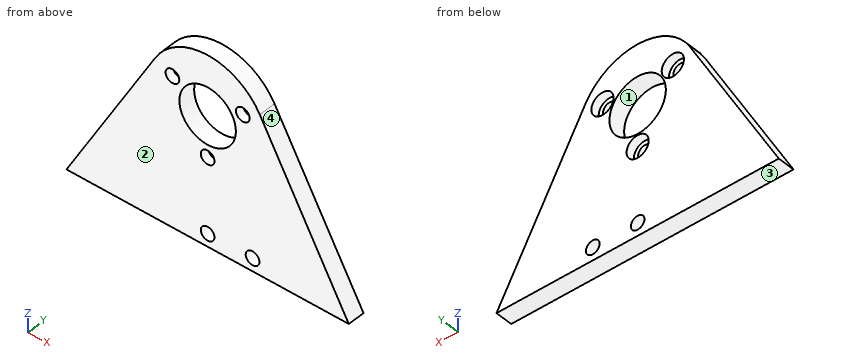
from build123d import *

# Parameters (mm, degrees)
EXTRUDE_1_DEPTH     = 4
SKETCH_3_R          = 1.6
SKETCH_3_R_2        = 6.6
CUT_EXTRUDE_3_DEPTH = 4
SKETCH_4_R          = 1.6
CUT_EXTRUDE_4_DEPTH = 4
SKETCH_5_R          = 2.6
CUT_EXTRUDE_6_DEPTH = 2


with BuildPart() as part:
    # 草图1 → 凸台-拉伸1 (new body)
    with BuildSketch(Plane(origin=(0, 0, 0), x_dir=(1, 0, 0), z_dir=(0, 1, 0))):
        with BuildLine():
            Line((33, 30), (12.193267422, -6.879260831))
            ThreePointArc((12.193267422, -6.879260831), (0, -14), (-12.193267422, -6.879260831))
            Line((-12.193267422, -6.879260831), (-33, 30))
            Line((-33, 30), (33, 30))
        make_face()
    extrude(amount=EXTRUDE_1_DEPTH)

    # 草图3 → 切除-拉伸3 (cut)
    with BuildSketch(Plane(origin=(0, 4, 0), x_dir=(1, 0, 0), z_dir=(0, 1, 0))):
        with Locations(Location((-8.227241336, -4.75, 0), (0, 0, 270))):
            Circle(SKETCH_3_R)
        with Locations(Location((8.227241336, -4.75, 0), (0, 0, 270))):
            Circle(SKETCH_3_R)
        with Locations(Location((0, 0, 0), (0, 0, 270))):
            Circle(SKETCH_3_R_2)
        with Locations(Location((0, 9.5, 0), (0, 0, 270))):
            Circle(SKETCH_3_R)
    extrude(amount=-CUT_EXTRUDE_3_DEPTH, mode=Mode.SUBTRACT)

    # 草图4 → 切除-拉伸4 (cut)
    with BuildSketch(Plane(origin=(0, 4, 0), x_dir=(1, 0, 0), z_dir=(0, 1, 0))):
        with Locations(Location((0, 27, 0), (0, 0, 270))):
            Circle(SKETCH_4_R)
        with Locations(Location((10.5, 27, 0), (0, 0, 270))):
            Circle(SKETCH_4_R)
    extrude(amount=-CUT_EXTRUDE_4_DEPTH, mode=Mode.SUBTRACT)

    # 草图5 → 切除-拉伸6 (cut)
    with BuildSketch(Plane(origin=(0, 4, 0), x_dir=(1, 0, 0), z_dir=(0, 1, 0))):
        with Locations(Location((0, 9.5, 0), (0, 0, 270))):
            Circle(SKETCH_5_R)
        with Locations(Location((8.227241336, -4.75, 0), (0, 0, 270))):
            Circle(SKETCH_5_R)
        with Locations(Location((-8.227241336, -4.75, 0), (0, 0, 270))):
            Circle(SKETCH_5_R)
    extrude(amount=-CUT_EXTRUDE_6_DEPTH, mode=Mode.SUBTRACT)


solid = part.part
Could you check a few things on this model? Use its own coordinates, in mm. Face numbers are marked on the shaded views. Give positions to 0.01 mm unless a question says otherwise; leave off trailing zeros. Write each loop counter-clockwise with the first axis right and the second up, starting at its lowest first coordinate (ties: lowest second). Pieces come first, ordered by that corner, then holes. Notation, with made-up numbers: (7.5, -27.5) -> (65.5, -27.5) arc R10 cw to (65.5, -12.5) -> close; hole circle Ø4 at (10, 18.25). An arc over 180 degrees is marked (long way). Write each question's results on one line, items separated by ' | '. Start each with the question number.
Q1. Suppose I cut it at D-D, the plane y = 2.7. List the corners of the cut face in (x, z) for me.
Q2. Suppose I cut it at A-A, the plane x = 0. List the corners of the cut face in (y, z) for me, and give its area (3 significant figures).
Q3. We'd pull the mould along Z, two halves only. Please class the marked faces 1, 2, 3 and 4: +Z half, -Z half, draft (parallel to the pull), parting line (faces both ways), or undercut.
Q4. I'm going to push flat-ended pins straight in: pin 1 Ø8 at (x, z) = (-6, -3.5) entering from -Y; pin 2 Ø4 at (x, z) = (-8.23, 4.75) entering from +Y; pin 3 Ø1.5 at (x, y) = (-10, 3.5) entering from +Z. Where does each tip first touch, or does it pass through?
Q5. Suppose I cut it at C-C, the plane z = -27. List the corners of the cut face in (x, y) for me.
Q6. Suppose I cut it at B-B, the plane z = -9.5. List the corners of the cut face in (x, y) for me, and give its area (3 significant figures).
Q7. I need wall thicknesses on probe 1 along Z at (x, y) = (-1, 2.05); probe 2 along Z at (x, y) = (0.5, 3.25); probe 3 along X at (y, z) = (3.45, 4.75). Which ranges of each line are inside material? Lowest first, please.
Outcome:
1) outline: (-33, -30) -> (33, -30) -> (12.19, 6.88) arc R14 ccw to (-12.19, 6.88) -> close; hole circle Ø5.2 at (-8.23, 4.75); hole circle Ø13.2 at (0, 0); hole circle Ø5.2 at (0, -9.5); hole circle Ø3.2 at (0, -27); hole circle Ø5.2 at (8.23, 4.75); hole circle Ø3.2 at (10.5, -27)
2) outline: (0, -30) -> (4, -30) -> (4, -28.6) -> (0, -28.6) -> close; (0, -25.4) -> (4, -25.4) -> (4, -12.1) -> (2, -12.1) -> (2, -11.1) -> (0, -11.1) -> close; (0, -7.9) -> (2, -7.9) -> (2, -6.9) -> (4, -6.9) -> (4, -6.6) -> (0, -6.6) -> close; (0, 6.6) -> (4, 6.6) -> (4, 14) -> (0, 14) -> close | area: 93.6 mm2
3) face 1: undercut | face 2: draft | face 3: -Z half | face 4: +Z half
4) pin 1: y = 0 | pin 2: y = 2 | pin 3: z = 10.51
5) outline: (-31.31, 0) -> (-1.6, 0) -> (-1.6, 4) -> (-31.31, 4) -> close; (1.6, 0) -> (8.9, 0) -> (8.9, 4) -> (1.6, 4) -> close; (12.1, 0) -> (31.31, 0) -> (31.31, 4) -> (12.1, 4) -> close
6) outline: (-21.43, 0) -> (-1.6, 0) -> (-1.6, 2) -> (-2.6, 2) -> (-2.6, 4) -> (-21.43, 4) -> close; (1.6, 0) -> (21.43, 0) -> (21.43, 4) -> (2.6, 4) -> (2.6, 2) -> (1.6, 2) -> close | area: 155 mm2
7) probe 1: -30 to -28.25, -25.75 to -11.9, -7.1 to -6.52, 6.52 to 13.96 | probe 2: -30 to -28.52, -25.48 to -12.05, -6.95 to -6.58, 6.58 to 13.99 | probe 3: -13.39 to -10.83, -5.63 to -4.58, 4.58 to 5.63, 10.83 to 13.39
